Read the model definition and answer for the solid it produces. Units are mm, in the model's axes. A direction names the side the tool comes from. Coordinates: 2 decimals unless noted, no trailing zeros. Write each loop counter-clockwise with the first axis right and the second up, starting at its lowest first coordinate (ties: lowest second). Pieces come first, ordered by that corner, then holes. Notation, with made-up numbers: (-34.75, -10) -> (10.25, -10) arc R28 ccw to (10.25, 24) -> close; hole circle Ø1 at (-8, 2.5). An arc over 180 degrees is marked (long way). One line per item, written item: value. Start each with the question number.
1. Find section C-C, the plane y = -21. Write down the section's boundary in (x, z).
2. For a pull along Z with two mould halves and no side action, classify faces 1 (the flat face through (-1, -2, -35)), 2 (the flat face through (-47, -55, -26)), 3 (the cylindrical face through (-50.474, -29.65, 27.109)) as pulls with the +Z half, pulls with the -Z half, needs draft (parallel to the pull), parting line crosses it, or undercut.
3. Find section B-B, the plane z = 20. Write down the section's boundary in (x, y).
4. Find section D-D, the plane x = 0. Write down the section's boundary in (y, z).
5. Find section A-A, the plane x = 42. Write down the section's boundary in (y, z), and give its area (3 significant figures).
6. Given P1, Ø0.8, axis at x = 0.5, z = 28, coming from the -Y side; P2, Ø3.5, axis at x = -28, z = -28, coming from the -Y side, each flat-ended and moving along its own axis, determine where each tip first touches the part or whether it passes through.
7. For faces 4 (the cylindrical face through (-27.94, -2.46, 26.6)), 5 (the flat face through (-48, -52, -28)), determine the directions among +Z, -Z, +X, -X, +Y, -Y from which every point of the face is accessible in a straight line to the end or side of a thin tool.
8. Consider line 1 along X through (y, z) = (-52.7, -27.5); line 2 along X through (y, z) = (-53, 27); line 3 along X through (y, z) = (-3.55, -28). Determine where each line is inside the solid, lowest interval first.
```python
from build123d import *

# Parameters (mm, degrees)
SKETCH1_W           = 110
SKETCH1_H           = 70
BOSS_EXTRUDE2_DEPTH = 5
SKETCH2_R           = 1.4
CUT_EXTRUDE1_DEPTH  = 5
SKETCH4_R           = 3
BOSS_EXTRUDE3_DEPTH = 50
SKETCH5_R           = 1.4
CUT_EXTRUDE2_DEPTH  = 3


with BuildPart() as part:
    # Sketch1 → Boss-Extrude2 (new body)
    with BuildSketch(Plane(origin=(0, 0, 0), x_dir=(1, 0, 0), z_dir=(0, 1, 0))):
        Rectangle(SKETCH1_W, SKETCH1_H)
    extrude(amount=-BOSS_EXTRUDE2_DEPTH)

    # Sketch2 → Cut-Extrude1 (cut)
    with BuildSketch(Plane(origin=(0, 0, 0), x_dir=(1, 0, 0), z_dir=(0, 1, 0))):
        with Locations(Location((-28, 28, 0), (0, 0, 270))):
            Circle(SKETCH2_R)
        with Locations(Location((42, 20, 0), (0, 0, 270))):
            Circle(SKETCH2_R)
        with Locations(Location((-28, -28, 0), (0, 0, 270))):
            Circle(SKETCH2_R)
        with Locations(Location((42, -20, 0), (0, 0, 270))):
            Circle(SKETCH2_R)
    extrude(amount=-CUT_EXTRUDE1_DEPTH, mode=Mode.SUBTRACT)

    # Sketch4 → Boss-Extrude3 (add)
    with BuildSketch(Plane.XZ.offset(5)):
        with Locations(Location((-47.5, 27.5, 0), (0, 0, 90))):
            Circle(SKETCH4_R)
        with Locations(Location((0, 27.5, 0), (0, 0, 90))):
            Circle(SKETCH4_R)
        with Locations(Location((0, -27.5, 0), (0, 0, 90))):
            Circle(SKETCH4_R)
        with Locations(Location((-47.5, -27.5, 0), (0, 0, 90))):
            Circle(SKETCH4_R)
    extrude(amount=BOSS_EXTRUDE3_DEPTH)

    # Sketch5 → Cut-Extrude2 (cut)
    with BuildSketch(Plane.XZ.offset(55)):
        with Locations(Location((-47.5, 27.5, 0), (0, 0, 270))):
            Circle(SKETCH5_R)
        with Locations(Location((0, 27.5, 0), (0, 0, 270))):
            Circle(SKETCH5_R)
        with Locations(Location((0, -27.5, 0), (0, 0, 90))):
            Circle(SKETCH5_R)
        with Locations(Location((-47.5, -27.5, 0), (0, 0, 90))):
            Circle(SKETCH5_R)
    extrude(amount=-CUT_EXTRUDE2_DEPTH, mode=Mode.SUBTRACT)


solid = part.part
```
Answer block:
1. outline: circle Ø6 at (-47.5, -27.5); circle Ø6 at (-47.5, 27.5); circle Ø6 at (0, -27.5); circle Ø6 at (0, 27.5)
2. face 1: pulls with the -Z half
2. face 2: needs draft
2. face 3: undercut
3. outline: (-55, -5) -> (40.6, -5) -> (40.6, 0) -> (-55, 0) -> close; (43.4, -5) -> (55, -5) -> (55, 0) -> (43.4, 0) -> close
4. outline: (-55, -30.5) -> (-5, -30.5) -> (-5, -35) -> (0, -35) -> (0, 35) -> (-5, 35) -> (-5, 30.5) -> (-55, 30.5) -> (-55, 28.9) -> (-52, 28.9) -> (-52, 26.1) -> (-55, 26.1) -> (-55, 24.5) -> (-5, 24.5) -> (-5, -24.5) -> (-55, -24.5) -> (-55, -26.1) -> (-52, -26.1) -> (-52, -28.9) -> (-55, -28.9) -> close
5. outline: (-5, -35) -> (0, -35) -> (0, -21.4) -> (-5, -21.4) -> close; (-5, -18.6) -> (0, -18.6) -> (0, 18.6) -> (-5, 18.6) -> close; (-5, 21.4) -> (0, 21.4) -> (0, 35) -> (-5, 35) -> close
5. area: 322 mm2
6. P1: stops at y = -52
6. P2: stops at y = -5
7. face 4: +Y, -Y
7. face 5: -Y
8. line 1: x = -50.5 to -48.9, -46.1 to -44.5, -3 to -1.4, 1.4 to 3
8. line 2: x = -50.46 to -48.81, -46.19 to -44.54, -2.96 to -1.31, 1.31 to 2.96
8. line 3: x = -55 to -29.4, -26.6 to 55
